Read the model definition and answer for the solid it produces. Units are mm, in the model's axes. A direction names the side the tool comes from. Give positions to 0.01 mm unless a question says otherwise; leave off trailing zeros. Loops run counter-clockwise (first coordinate to the right, second up) from the corner with the lowest first, then second, coordinate; pieces in that order, holes last. Notation, with made-up numbers: (5.5, -8) - (16.5, -8) arc R33 cw to (16.5, 20) - close; hole circle Ø7 at (9, 47). An arc over 180 degrees is marked (long way). Put each result on its own line as item: value. Start each with the question number.
1. A cutting plane is placed at B-B, the plane y = 2.75. Determine the outline of the cut face in (x, z).
2. For faces 4 (the flat face through (-4.6, -4.2, 3.5)), 5 (the flat face through (-0.402, 3.823, 2.993)), determine the directions among +Z, -Z, +X, -X, +Y, -Y from which every point of the face is accessible in a straight line to the end or side of a thin tool.
3. Consider L1, parallel to X at y = -0.75, z = 0.85; L2, parallel to Y at x = -7.5, z = 0.25; L3, parallel to Z at x = 27, y = -2.25. Determine where each line is inside the solid, lowest interval first. Write a range as from..to.
4. A cutting plane is placed at C-C, the plane x = 5.5. Determine the outline of the cut face in (y, z), plus the area to 3 significant figures.
5. For a pull along X with two mould halves and no side action, classify faces 1 (the flat face through (0, 0, 0)), 2 (the flat face through (30.5, 0, 1)), 3 (the flat face through (-30.5, 0, 1)) as released by +X, released by -X, zero draft, split by the parting line, or undercut.
6. A cutting plane is placed at A-A, the plane z = 1.95. Determine the outline of the cut face in (x, y).
7. Given pin 1 Ø2 at (x, y) = (12, -0.5) entering from +Z, flat-ended and moving along its own axis, determine where the tip first touches the part or whether it passes through.
```python
from build123d import *

# Parameters (mm, degrees)
SKETCH002_W      = 61
SKETCH002_H      = 11.4
SKETCH002_W_2    = 57
SKETCH002_H_2    = 7.4
PAD002_DEPTH     = 3.5
SKETCH003_W      = 61
SKETCH003_H      = 11.4
PAD003_DEPTH     = 2
CHAMFER001_SIZE2 = 1
CHAMFER001_SIZE  = 0.25
FILLET_R         = 0.5


with BuildPart() as part:
    # Sketch002 → Pad002 (new body)
    with BuildSketch(Plane.XY):
        Rectangle(SKETCH002_W, SKETCH002_H)
        Rectangle(SKETCH002_W_2, SKETCH002_H_2, mode=Mode.SUBTRACT)
    extrude(amount=PAD002_DEPTH)

    # Sketch003 (on Face9 of Pad002) → Pad003 (join)
    with BuildSketch(Plane(origin=(0, 0, 0), x_dir=(1, 0, 0), z_dir=(0, 0, -1))):
        Rectangle(SKETCH003_W, SKETCH003_H)
    extrude(amount=PAD003_DEPTH)

    # Chamfer001
    chamfer001_edges = [part.edges().sort_by_distance(p)[0] for p in [
        (0, 3.7, 3.5),
        (-28.5, 0, 3.5),
        (0, -3.7, 3.5),
        (28.5, 0, 3.5),
    ]]
    chamfer001_side = part.faces().sort_by_distance((29.879439, 0, 3.5))[0]
    chamfer(chamfer001_edges, length=CHAMFER001_SIZE, length2=CHAMFER001_SIZE2, reference=chamfer001_side)

    # Fillet
    fillet_edges = [part.edges().sort_by_distance(p)[0] for p in [
        (30.5, -5.7, 0.75),
        (30.5, 0, -2),
        (30.5, 5.7, 0.75),
        (30.5, 0, 3.5),
        (-30.5, -5.7, 0.75),
        (0, -5.7, -2),
        (0, -5.7, 3.5),
        (-30.5, 5.7, 0.75),
        (-30.5, 0, -2),
        (-30.5, 0, 3.5),
        (0, 5.7, -2),
        (0, 5.7, 3.5),
    ]]
    fillet(fillet_edges, radius=FILLET_R)


solid = part.part
```
Return value:
1. outline: (-30.5, -1.5) arc R0.5 ccw to (-30, -2) - (30, -2) arc R0.5 ccw to (30.5, -1.5) - (30.5, 3) arc R0.5 ccw to (30, 3.5) - (28.75, 3.5) - (28.5, 2.5) - (28.5, 0) - (-28.5, 0) - (-28.5, 2.5) - (-28.75, 3.5) - (-30, 3.5) arc R0.5 ccw to (-30.5, 3) - close
2. face 4: +Z, +X, -X, +Y, -Y
2. face 5: +Z
3. L1: x = -30.5..-28.5, 28.5..30.5
3. L2: y = -5.7..-3.7, 3.7..5.7
3. L3: z = -2..0
4. outline: (-5.7, -1.5) arc R0.5 ccw to (-5.2, -2) - (5.2, -2) arc R0.5 ccw to (5.7, -1.5) - (5.7, 3) arc R0.5 ccw to (5.2, 3.5) - (3.95, 3.5) - (3.7, 2.5) - (3.7, 0) - (-3.7, 0) - (-3.7, 2.5) - (-3.95, 3.5) - (-5.2, 3.5) arc R0.5 ccw to (-5.7, 3) - close
4. area: 36.3 mm2
5. face 1: undercut
5. face 2: released by +X
5. face 3: released by -X
6. outline: (-30.5, -5.2) arc R0.5 ccw to (-30, -5.7) - (30, -5.7) arc R0.5 ccw to (30.5, -5.2) - (30.5, 5.2) arc R0.5 ccw to (30, 5.7) - (-30, 5.7) arc R0.5 ccw to (-30.5, 5.2) - close; hole (-28.5, -3.7) - (28.5, -3.7) - (28.5, 3.7) - (-28.5, 3.7) - close
7. pin 1: stops at z = 0
